Design review of the part built by this model. Coordinates are the model's own, in mm. A direction names the side the tool comes from. Round coordinates to 2 decimals unless told otherwise and drop trailing zeros. Loops run counter-clockwise (first coordinate to the right, second up) from the corner with the lowest first, then second, coordinate; pieces in that order, holes last. Notation, with made-up numbers: M 87.25,54.25 L 114.25,54.25 A27 ccw 114.25,86.25 Z; hole C 84,-29.75 d3. An arc over 180 degrees is marked long. One line per item, written item: value. Start each with the question number.
Item 1: Mouldability with a two-part tool opening along Z and no side actions: class faces 1 (the flat face through (2, 89.789, 0)), 2 (the cylindrical face through (1.48, 57.02, -0.29)), 3 (the cylindrical face through (1.48, 3.89, -15.41)) as released by +Z, released by -Z, zero draft, split by the parting line, or undercut.
Item 2: Clearance check with flat-ended pins moving along their axes: pin 1 (3.5 mm diameter, centred on y = 0, z = 0, fed in from +X); pin 2 (1 mm diameter, centred on x = 2, z = 6.5, fed in from -Y); pin 3 (0.9 mm diameter, centred on x = 1, y = 63.5, fed in from +Z). State where each tip first meets the part, or that it passes through.
Item 3: For faces 4 (the cylindrical face through (1.48, -15.41, -3.89)), 5 (the cylindrical face through (1.479, 8.153, -13.677)), 6 (the cylindrical face through (1.479, 0.807, -15.87)), list the 3-axis set-ups (+Z, -Z, +X, -X, +Y, -Y) from which the entire face can be reached by the end or side of a thin tool; tool diameter is ignored.
Item 4: For line 1 along Z through (x, y) = (1.3, 80); line 2 along Z through (x, y) = (2.15, 46); line 3 along Y through (x, z) = (1.2, -15), list the stretches that pass through material, from the lowest coordinate up.
Item 5: We need section A-A (y = 37.5). Write out the cut boundary in (x, z).
Item 6: We need section B-B (x = 1.4). State how many separate pieces and enclosed holes the cut face has, then the cut area to 3 significant figures.
from build123d import *

# Parameters (mm, degrees)
BASPROSKE_W          = 3
BASPROSKE_H          = 17
TOOTHCUT_DEPTH       = 25.228082879
TEETHCUTS_COUNT      = 32
TEETHCUTS_ANGLE      = 348.75
BORSKE_R             = 2
BORE_DEPTH           = 50.0000508
SKETCH1_W            = 15
SKETCH1_H            = 80
BOSS_EXTRUDE1_DEPTH  = 3
M4_CLEARANCE_HOLE1_D = 4.5
M2_CLEARANCE_HOLE1_D = 2.4


with BuildPart() as part:
    # BasProSke → Base-Revolve (revolve)
    with BuildSketch(Plane(origin=(0, 0, 0), x_dir=(1, 0, 0), z_dir=(0, 1, 0)), mode=Mode.PRIVATE) as base_revolve_sk:
        with Locations((1.5, 8.5)):
            Rectangle(BASPROSKE_W, BASPROSKE_H)
    revolve(base_revolve_sk.sketch.rotate(Axis((-10, 0, 0), (1, 0, 0)), 180), axis=Axis((-10, 0, 0), (1, 0, 0)))

    # TooCutSke → ToothCut (cut, through all)
    with BuildSketch(Plane(origin=(0, 0, 0), x_dir=(0, 0, -1), z_dir=(1, 0, 0))):
        with BuildLine():
            ThreePointArc((0.462036907, 14.741761187), (0, 14.749), (-0.462036907, 14.741761187))
            ThreePointArc((-0.462036907, 14.741761187), (-0.81854142, 15.899240468), (-1.386721275, 16.9688317))
            ThreePointArc((-1.386721275, 16.9688317), (0, 17.0254), (1.386721275, 16.9688317))
            ThreePointArc((1.386721275, 16.9688317), (0.81854142, 15.899240468), (0.462036907, 14.741761187))
        make_face()
    toothcut = extrude(amount=TOOTHCUT_DEPTH, mode=Mode.SUBTRACT)

    # TeethCuts: ToothCut ×32 about axis
    teethcuts_axis = Axis((-10, 0, 0), (1, 0, 0))
    for i in range(1, TEETHCUTS_COUNT):
        add(toothcut.rotate(teethcuts_axis, i * TEETHCUTS_ANGLE / (TEETHCUTS_COUNT - 1)), mode=Mode.SUBTRACT)

    # BorSke → Bore (cut, symmetric)
    with BuildSketch(Plane(origin=(0, 0, 0), x_dir=(0, 0, -1), z_dir=(1, 0, 0))):
        with Locations(Location((0, 0, 0), (0, 0, 180))):
            Circle(BORSKE_R)
    extrude(amount=BORE_DEPTH, both=True, mode=Mode.SUBTRACT)

    # Sketch1 → Boss-Extrude1 (add)
    with BuildSketch(Plane(origin=(3, 0, 0), x_dir=(0, 0, -1), z_dir=(1, 0, 0))):
        with Locations((0, 49.788617333)):
            Rectangle(SKETCH1_W, SKETCH1_H)
    extrude(amount=-BOSS_EXTRUDE1_DEPTH)

    # M4 Clearance Hole1 (through all)
    with Locations(Plane(origin=(3, 0, 0), x_dir=(0, 0, -1), z_dir=(1, 0, 0))):
        with Locations((0, 79.788617333), (0, 29.788617333), (0, 54.788617333), (0, 0)):
            Hole(M4_CLEARANCE_HOLE1_D / 2)

    # M2 Clearance Hole1 (through all)
    with Locations(Plane(origin=(3, 0, 0), x_dir=(0, 0, -1), z_dir=(1, 0, 0))):
        with Locations((0, 7.5), (0, -7.5)):
            Hole(M2_CLEARANCE_HOLE1_D / 2)


solid = part.part
A:
1. face 1: zero draft
1. face 2: undercut
1. face 3: released by -Z
2. pin 1: through
2. pin 2: y = -14.53
2. pin 3: z = 7.5
3. face 4: +X, -X, -Y
3. face 5: +X, -X
3. face 6: -Z, +X, -X
4. line 1: -7.5 to -2.24, 2.24 to 7.5
4. line 2: -7.5 to 7.5
4. line 3: -8 to -7.57, -5.33 to -3.64, -2.4 to -0.52, 0.52 to 2.4, 3.64 to 5.33, 7.57 to 8
5. outline: M 0,-7.5 L 3,-7.5 L 3,7.5 L 0,7.5 Z
6. separate pieces: 1
6. enclosed holes: 6
6. area: 1,830 mm2
